```python
from build123d import *

# Parameters (mm, degrees)
SKETCH1_W           = 60.5
SKETCH1_H           = 9.5
SKETCH1_R           = 0.4
BOSS_EXTRUDE1_DEPTH = 6.5
SKETCH2_R           = 1
BOSS_EXTRUDE2_DEPTH = 3.5
SKETCH2_3_R         = 0.6
BOSS_EXTRUDE3_DEPTH = 5
SKETCH4_W           = 55
SKETCH4_H           = 2.5
CUT_EXTRUDE1_DEPTH  = 1
FILLET1_R           = 1


with BuildPart() as part:
    # Sketch1 → Boss-Extrude1 (new body)
    with BuildSketch(Plane(origin=(0, 0, 0), x_dir=(1, 0, 0), z_dir=(0, 1, 0))):
        Rectangle(SKETCH1_W, SKETCH1_H)
        with Locations(Location((-28, 0, 0), (0, 0, 270))):
            Circle(SKETCH1_R, mode=Mode.SUBTRACT)
        with Locations(Location((28, 0, 0), (0, 0, 270))):
            Circle(SKETCH1_R, mode=Mode.SUBTRACT)
    extrude(amount=BOSS_EXTRUDE1_DEPTH)

    # Sketch2 → Boss-Extrude2 (add)
    with BuildSketch(Plane.XZ):
        with Locations(Location((-25.1, 4.25, 0), (0, 0, 150))):
            Circle(SKETCH2_R)
        with Locations(Location((-23.9, -4.25, 0), (0, 0, 210))):
            Circle(SKETCH2_R)
        with Locations(Location((25.1, 4.25, 0), (0, 0, 30))):
            Circle(SKETCH2_R)
        with Locations(Location((23.9, -4.25, 0), (0, 0, 330))):
            Circle(SKETCH2_R)
    extrude(amount=BOSS_EXTRUDE2_DEPTH)

    # Sketch2_3 → Boss-Extrude3 (add)
    with BuildSketch(Plane.XZ):
        with Locations(Location((-29.25, 1.75, 0), (0, 0, 90))):
            Circle(SKETCH2_3_R)
        with Locations(Location((-29.25, -1.75, 0), (0, 0, 90))):
            Circle(SKETCH2_3_R)
        with Locations(Location((29.25, -1.75, 0), (0, 0, 90))):
            Circle(SKETCH2_3_R)
    extrude(amount=BOSS_EXTRUDE3_DEPTH)

    # Sketch4 → Cut-Extrude1 (cut)
    with BuildSketch(Plane(origin=(0, 6.5, 0), x_dir=(1, 0, 0), z_dir=(0, 1, 0))):
        Rectangle(SKETCH4_W, SKETCH4_H)
    extrude(amount=-CUT_EXTRUDE1_DEPTH, mode=Mode.SUBTRACT)

    # Fillet1
    fillet1_edges = [part.edges().sort_by_distance(p)[0] for p in [
        (30.25, 6.5, 0),
        (0, 6.5, -4.75),
        (-30.25, 6.5, 0),
        (0, 6.5, 4.75),
    ]]
    fillet(fillet1_edges, radius=FILLET1_R)


solid = part.part
```
Can you work these out from the model? Positions are in its coordinate system, mm. A direction names the side the tool comes from. Give positions to 0.01 mm unless a question says otherwise; leave off trailing zeros. Order: outer loops, then holes, each group sorted by start corner. A loop starts at its lowest first (then second) coordinate and runs counter-clockwise, first axis right, second up. Notation, with made-up numbers: M -37,58.25 L 17,58.25 A18 ccw 17,67.25 Z; hole C 79.25,-0.75 d6. An arc over 180 degrees is marked long. Write item = value, one per line. Start each with the question number.
Q1. Suppose I cut it at A-A (y = -1.25). Write out the boundary of the cut face in (x, z), plus the area to 3 significant figures.
Q2. Suppose I cut it at D-D (z = -1.75). Write out the boundary of the cut face in (x, y).
Q3. Will these pins go through, and if not, where does the flat tip stop? pin 1 Ø4.5 at (x, y) = (15, 2.5) entering from -Z; pin 2 Ø1 at (x, z) = (-24, -4) entering from -Y; pin 3 Ø6 at (x, y) = (8.5, 1) entering from +Z.
Q4. For faces 1 (the flat face through (0, 6, 1.25)), 2 (the flat face through (-29, -5, 2)), 3 (the cylindrical face through (-29.845, -2.465, -1.828)), which set-ups out of +Z, -Z, +X, -X, +Y, -Y let a thin tool reach every point of the face, with its end or its side?
Q5. We'd pull the mould along Z, two halves only. Please class faces 4 (the flat face through (29, -5, -2)), 5 (the cylindrical face through (0.424, 6.199, -4.465)), 6 (the cylindrical face through (24.49, -1.73, 5.04)): pulls with the +Z half, pulls with the -Z half, needs draft (parallel to the pull), parting line crosses it, or undercut.
Q6. Suppose I cut it at C-C (y = 2). Write out the boundary of the cut face in (x, z), plus the area to 3 significant figures.
Q7. Suppose I cut it at B-B (x = 14). Write out the boundary of the cut face in (y, z).
Q8. I need wall thicknesses on probe 1 along X at (y, z) = (4.5, 0); probe 2 along Z at (x, y) = (-28, 5). Which ranges of each line are inside material? Lowest first, please. Write a range as [from, to].
Check result:
q1.outline = C -29.25,-1.75 d1.2; C -29.25,1.75 d1.2; C -25.1,4.25 d2; C -23.9,-4.25 d2; C 23.9,-4.25 d2; C 25.1,4.25 d2; C 29.25,-1.75 d1.2
q1.area = 16.0 mm2
q2.outline = M -30.25,0 L -29.85,0 L -29.85,-5 L -28.65,-5 L -28.65,0 L 28.65,0 L 28.65,-5 L 29.85,-5 L 29.85,0 L 30.25,0 L 30.25,5.5 A1 ccw 29.25,6.5 L -29.25,6.5 A1 ccw -30.25,5.5 Z
q3.pin_1 = -4.75
q3.pin_2 = -3.5
q3.pin_3 = 4.75
q4.face_1 = +Y
q4.face_2 = +Z, -Z, +X, -X, -Y
q4.face_3 = -Y
q5.face_4 = needs draft
q5.face_5 = pulls with the -Z half
q5.face_6 = undercut
q6.outline = M -30.25,-4.75 L 30.25,-4.75 L 30.25,4.75 L -30.25,4.75 Z; hole C -28,0 d0.8; hole C 28,0 d0.8
q6.area = 574 mm2
q7.outline = M 0,-4.75 L 5.5,-4.75 A1 ccw 6.5,-3.75 L 6.5,-1.25 L 5.5,-1.25 L 5.5,1.25 L 6.5,1.25 L 6.5,3.75 A1 ccw 5.5,4.75 L 0,4.75 Z
q8.probe_1 = [-30.25, -28.4], [-27.6, 27.6], [28.4, 30.25]
q8.probe_2 = [-4.75, -0.4], [0.4, 4.75]
